from build123d import *

# Parameters (mm, degrees)
SKETCH1_R                    = 3.175
BOSS_EXTRUDE1_DEPTH          = 9.525
SKETCH2_W                    = 12.7
SKETCH2_H                    = 15.875
CUT_EXTRUDE1_DEPTH           = 7.35
CUT_EXTRUDE1_DEPTH_BACK      = 7.35
F_1_8_0_125_DIAMETER_HOLE1_D = 3.175
FILLET2_R                    = 3.175
CHAMFER1_SIZE                = 0.508


with BuildPart() as part:
    # Sketch1 → Boss-Extrude1 (new body, symmetric)
    with BuildSketch(Plane.XY):
        with BuildLine():
            Line((-6.35, 0), (-6.35, -12.7))
            Line((-6.35, -12.7), (6.35, -12.7))
            Line((6.35, -12.7), (6.35, 0))
            ThreePointArc((6.35, 0), (0, 6.35), (-6.35, 0))
        make_face()
        Circle(SKETCH1_R, mode=Mode.SUBTRACT)
    extrude(amount=BOSS_EXTRUDE1_DEPTH, both=True)

    # Sketch2 → Cut-Extrude1 (cut, two sides)
    with BuildSketch(Plane(origin=(0, 0, 0), x_dir=(0, 0, -1), z_dir=(1, 0, 0))) as cut_extrude1_sk:
        with Locations((0, -1.5875)):
            Rectangle(SKETCH2_W, SKETCH2_H)
    extrude(amount=CUT_EXTRUDE1_DEPTH, mode=Mode.SUBTRACT)
    extrude(cut_extrude1_sk.sketch, amount=-CUT_EXTRUDE1_DEPTH_BACK, mode=Mode.SUBTRACT)

    # 1/8 (0.125) Diameter Hole1 (through all)
    with Locations(Plane(origin=(0, -9.525, 0), x_dir=(1, 0, 0), z_dir=(0, 1, 0))):
        with Locations((-3.175, 0), (3.175, 0)):
            Hole(F_1_8_0_125_DIAMETER_HOLE1_D / 2)

    # Fillet2
    fillet2_edges = [part.edges().sort_by_distance(p)[0] for p in [
        (0, -9.525, 6.35),
        (0, -9.525, -6.35),
    ]]
    fillet(fillet2_edges, radius=FILLET2_R)

    # Chamfer1
    chamfer1_edges = [part.edges().sort_by_distance(p)[0] for p in [
        (-6.35, -6.35, 9.525),
        (-3.175, 0, -9.525),
        (-3.175, 0, 9.525),
        (0, -12.7, 9.525),
        (0, 6.35, 6.35),
        (-6.35, -3.175, 6.35),
        (-3.175, 0, 6.35),
        (-3.175, 0, -6.35),
        (6.35, -3.175, -6.35),
        (0, 6.35, -6.35),
        (-6.35, -3.175, -6.35),
        (6.35, -3.175, 6.35),
        (6.35, -6.35, 9.525),
        (0, -12.7, -9.525),
        (4.7625, -9.525, 0),
        (4.7625, -12.7, 0),
        (-6.35, -6.35, -9.525),
        (-1.5875, -9.525, 0),
        (-1.5875, -12.7, 0),
        (0, 6.35, -9.525),
        (-6.35, -9.525, 0),
        (6.35, -9.525, 0),
        (6.35, -6.35, -9.525),
        (6.35, -8.59506403, -5.42006403),
        (-6.35, -8.59506403, -5.42006403),
        (6.35, -8.59506403, 5.42006403),
        (-6.35, -8.59506403, 5.42006403),
        (0, 6.35, 9.525),
        (6.35, -12.7, 0),
        (-6.35, -12.7, 0),
    ]]
    chamfer(chamfer1_edges, length=CHAMFER1_SIZE)


solid = part.part
Verification items for the finished model (mm, model axes). A direction names the side the tool comes from. Round coordinates to 2 decimals unless told otherwise and drop trailing zeros.
(1) Depth check by flat-ended pin: pin 1 Ø2 at (y, z) = (2, -7.5) entering from -X; pin 2 Ø7 at (x, z) = (0, 1) entering from +Y. Enter the tip coordinate at first touch or a pass-through.
Returned:
pin 1: stops at x = -6.27
pin 2: stops at y = -9.24
(2) Mould release check, pull along Z, two halves, no side actions. Record for faces 6 (the cylindrical face through (0.082, -8.57, -5.445)), 7 (the cylindrical face through (0.14, 6.35, -7.92)), 8 (the conical face through (0.131, 5.978, -9.387)), 9 (the conical face through (0.132, 5.985, -6.495)): pulls with the +Z half, pulls with the -Z half, needs draft (parallel to the pull), parting line crosses it, or undercut.
Returned:
face 6: undercut
face 7: needs draft
face 8: pulls with the -Z half
face 9: undercut
(3) Material ranges on line 1 (X direction, y = -11.6, z = 0); line 2 (Z direction, x = -4.5, y = -4) (3 decimals), recorded low to high.
Returned:
line 1: x = -6.35 to -4.76, -1.59 to 1.59, 4.76 to 6.35
line 2: z = -9.525 to -6.35, 6.35 to 9.525
(4) Section check A-A (z = 0). Give the number of separate pieces and of enclosed holes in the cut face, plus the area to 3 significant figures.
Returned:
separate pieces: 3
enclosed holes: 0
area: 18.6 mm2
(5) Access from +Z, -Z, +X, -X, +Y, -Y to the whole of each face (thin tool, end or side, straight path). Record for faces 1 (the conical face through (5.987, -8.723, -5.496)), 2 (the conical face through (-5.987, -8.671, -5.548)), 3 (the flat face through (0, -9.525, 0)), 4 (the cylindrical face through (-0.69, -3.1, 7.92)), 5 (the cylindrical face through (1.66, -11.13, -0.48)).
Returned:
face 1: +X, +Y
face 2: -X, +Y
face 3: +X, -X, +Y
face 4: +Z, -Z
face 5: +Y, -Y
